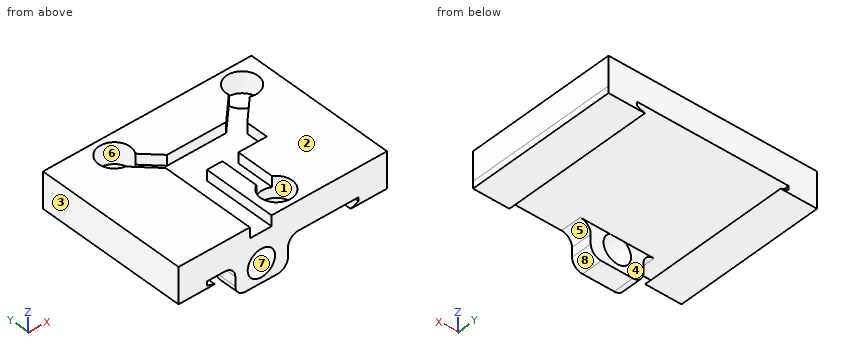
Autodesk Inventor part; units mm, degrees
ref_plane "YZ Plane" through (0, 0, 0) normal (1, 0, 0) x (0, 1, 0)
ref_plane "XZ Plane" through (0, 0, 0) normal (0, 1, 0) x (-1, 0, 0)
ref_plane "XY Plane" through (0, 0, 0) normal (0, 0, 1) x (1, 0, 0)
ref_plane "Work Plane1" through (52.5141, 202.7033, 6.4479) normal (0, 0, -1) x (0, 1, 0)
sketch "Sketch1" plane through (52.5141, 202.7033, 6.4479) normal (0, 0, -1) x (0, 1, 0)
  circle A0 centre (-59.8114, -30.5) radius 1.4 construction
  circle A1 centre (-38.8114, -18.3756) radius 1.4
  circle A2 centre (-38.8114, -42.6244) radius 1.4 construction
  circle A3 centre (41, 0) radius 1.65
  circle A4 centre (-9, 0) radius 1.65
  circle A5 centre (-9, 50) radius 1.65
  circle A6 centre (41, 50) radius 1.65
  circle A7 centre (16, 50) radius 1.65
  circle A8 centre (-9, 25) radius 1.65
  circle A9 centre (16, 0) radius 1.65
  circle A10 centre (41, 25) radius 1.65
  line L0 (80, 55) -> (-80, 55)
  line L1 (-80, 55) -> (-80, -55)
  line L2 (-80, -55) -> (80, -55)
  line L3 (80, -55) -> (80, 55)
  line L4 (-36.5, 0) -> (-36.5, -50)
  line L5 (-14, 0) -> (-36.5, 0)
  line L6 (-14, -5) -> (-14, 0)
  line L7 (72, -5) -> (-14, -5)
  line L8 (72, -50) -> (72, -5)
  line L9 (-36.5, -50) -> (72, -50)
  line L10 (-4, 45) -> (-4, 5)
  line L11 (36, 45) -> (-4, 45)
  line L12 (36, 5) -> (36, 45)
  line L13 (-4, 5) -> (36, 5)
  line L14 (-64.5989, -17.0433) -> (-64.5989, -57.0433) construction
  line L15 (-64.5989, -57.0433) -> (-34.5989, -57.0433) construction
  line L16 (-34.5989, -57.0433) -> (-34.5989, -17.0433) construction
  line L17 (-34.5989, -17.0433) -> (-64.5989, -17.0433) construction
  line L18 (-34.8114, -13.0433) -> (-63.8114, -13.0433)
  line L19 (-63.8114, -13.0433) -> (-63.8114, -52.6244)
  line L20 (-63.8114, -52.6244) -> (-34.8114, -52.6244)
  line L21 (-34.8114, -52.6244) -> (-34.8114, -13.0433)
  circle A11 centre (-59.8114, -30.5) radius 3
  circle A12 centre (-38.8114, -18.3756) radius 3
  circle A13 centre (-38.8114, -42.6244) radius 3 construction
  line L22 (-36.5, -35.1157) -> (-41.75, -35.1157) construction
  line L23 (-41.75, -35.1157) -> (-41.75, -38.5657) construction
  line L24 (-41.75, -38.5657) -> (-56.86, -38.5657) construction
  line L25 (-56.86, -38.5657) -> (-56.86, -35.1157) construction
  line L26 (-56.86, -35.1157) -> (-60.26, -35.1157) construction
  line L27 (-60.26, -35.1157) -> (-60.26, -52.0657) construction
  line L28 (-60.26, -52.0657) -> (-36.5, -52.0657) construction
  line L29 (-36.5, -52.0657) -> (-36.5, -35.1157) construction
  line L30 (-41.75, -28.3657) -> (-36.5, -28.3657) construction
  line L31 (-36.5, -28.3657) -> (-36.5, -25.0657) construction
  line L32 (-36.5, -25.0657) -> (-60.26, -25.0657) construction
  line L33 (-60.26, -25.0657) -> (-60.26, -28.3657) construction
  line L34 (-60.26, -28.3657) -> (-56.86, -28.3657) construction
  line L35 (-56.86, -28.3657) -> (-56.86, -27.0942) construction
  line L36 (-56.86, -27.0942) -> (-41.75, -27.0942) construction
  line L37 (-41.75, -27.0942) -> (-41.75, -28.3657) construction
  line L38 (-56.86, -35.1157) -> (-60.26, -35.1157) construction
  line L39 (-56.86, -38.5657) -> (-56.86, -35.1157) construction
  line L40 (-41.75, -38.5657) -> (-56.86, -38.5657) construction
  line L41 (-41.75, -35.1157) -> (-41.75, -38.5657) construction
  line L42 (-36.5, -35.1157) -> (-41.75, -35.1157) construction
  line L43 (-36.5, -35.05) -> (-36.5, -35.1157) construction
  line L44 (-36.5, -35.05) -> (-56.86, -35.05) construction
  line L45 (-36.5, -34.78) -> (-36.5, -35.05) construction
  line L46 (-36.5, -34.78) -> (-56.86, -34.78) construction
  line L47 (-36.5, -34.51) -> (-36.5, -34.78) construction
  line L48 (-36.5, -34.51) -> (-56.86, -34.51) construction
  line L49 (-36.5, -34.24) -> (-36.5, -34.51) construction
  line L50 (-36.5, -34.24) -> (-56.86, -34.24) construction
  line L51 (-36.5, -33.97) -> (-36.5, -34.24) construction
  line L52 (-36.5, -33.97) -> (-56.86, -33.97) construction
  line L53 (-36.5, -33.7) -> (-36.5, -33.97) construction
  line L54 (-36.5, -33.7) -> (-56.86, -33.7) construction
  line L55 (-36.5, -33.43) -> (-36.5, -33.7) construction
  line L56 (-36.5, -33.43) -> (-56.86, -33.43) construction
  line L57 (-36.5, -33.16) -> (-36.5, -33.43) construction
  line L58 (-36.5, -33.16) -> (-56.86, -33.16) construction
  line L59 (-36.5, -32.89) -> (-36.5, -33.16) construction
  line L60 (-36.5, -32.89) -> (-56.86, -32.89) construction
  line L61 (-36.5, -32.62) -> (-36.5, -32.89) construction
  line L62 (-36.5, -32.62) -> (-56.86, -32.62) construction
  line L63 (-36.5, -32.35) -> (-36.5, -32.62) construction
  line L64 (-36.5, -32.35) -> (-56.86, -32.35) construction
  line L65 (-36.5, -32.08) -> (-36.5, -32.35) construction
  line L66 (-36.5, -32.08) -> (-56.86, -32.08) construction
  line L67 (-36.5, -31.81) -> (-36.5, -32.08) construction
  line L68 (-36.5, -31.81) -> (-56.86, -31.81) construction
  line L69 (-36.5, -31.54) -> (-36.5, -31.81) construction
  line L70 (-36.5, -31.54) -> (-56.86, -31.54) construction
  line L71 (-36.5, -31.27) -> (-36.5, -31.54) construction
  line L72 (-36.5, -31.27) -> (-56.86, -31.27) construction
  line L73 (-36.5, -31) -> (-36.5, -31.27) construction
  line L74 (-36.5, -31) -> (-56.86, -31) construction
  line L75 (-36.5, -30.73) -> (-36.5, -31) construction
  line L76 (-36.5, -30.73) -> (-56.86, -30.73) construction
  line L77 (-36.5, -30.46) -> (-36.5, -30.73) construction
  line L78 (-36.5, -30.46) -> (-56.86, -30.46) construction
  line L79 (-36.5, -30.19) -> (-36.5, -30.46) construction
  line L80 (-36.5, -30.19) -> (-56.86, -30.19) construction
  line L81 (-36.5, -29.92) -> (-36.5, -30.19) construction
  line L82 (-36.5, -29.92) -> (-56.86, -29.92) construction
  line L83 (-36.5, -29.65) -> (-36.5, -29.92) construction
  line L84 (-36.5, -29.65) -> (-56.86, -29.65) construction
  line L85 (-36.5, -29.38) -> (-36.5, -29.65) construction
  line L86 (-36.5, -29.38) -> (-56.86, -29.38) construction
  line L87 (-36.5, -29.11) -> (-36.5, -29.38) construction
  line L88 (-36.5, -29.11) -> (-56.86, -29.11) construction
  line L89 (-36.5, -28.84) -> (-36.5, -29.11) construction
  line L90 (-36.5, -28.84) -> (-56.86, -28.84) construction
  line L91 (-36.5, -28.3657) -> (-36.5, -28.84) construction
  line L92 (-41.75, -28.3657) -> (-36.5, -28.3657) construction
  line L93 (-41.75, -27.0942) -> (-41.75, -28.3657) construction
  line L94 (-56.86, -27.0942) -> (-41.75, -27.0942) construction
  line L95 (-56.86, -28.3657) -> (-56.86, -27.0942) construction
  line L96 (-60.26, -28.3657) -> (-56.86, -28.3657) construction
  line L97 (-60.26, -35.1157) -> (-60.26, -28.3657) construction
  line L98 (-60.26, -25.0657) -> (-36.5, -25.0657) construction
  line L99 (-36.5, -25.0657) -> (-36.5, -52.0657) construction
  line L100 (-60.26, -52.0657) -> (-60.26, -25.0657) construction
  line L101 (-57.1632, -22.5233) -> (-33.4032, -22.5233) construction
  line L102 (-33.4032, -22.5233) -> (-33.4032, -49.5233) construction
  line L103 (-33.4032, -49.5233) -> (-57.1632, -49.5233) construction
  line L104 (-57.1632, -49.5233) -> (-57.1632, -22.5233) construction
  circle A14 centre (-38.8114, -42.6244) radius 3
  point P0 (-202.7033, -52.5141)
  point P1 (-56.7146, -27.9576)
  dimension "d0" = 4
  dimension "d2" = 4
  dimension "d3" = 4
  dimension "d4" = 6
  dimension "d5" = 6
  dimension "d6" = 6
  dimension "d10" = 10
extrude "Extrusion1" add sketch "Sketch1" along normal blind 4 contours L18 L21 L9 L4 A14 A12 | L4 A12 A14 L9 L21 L20 L19 L18
sketch "Sketch2" plane through (52.5141, 202.7033, 2.4479) normal (0, 0, -1) x (-1, 0, 0)
  circle A0 centre (42.6244, -38.8114) radius 3
  circle A1 centre (18.3756, -38.8114) radius 3
  circle A2 centre (30.5, -59.8114) radius 3
  line L0 (13.0433, -34.8114) -> (13.0433, -63.8114)
  line L1 (13.0433, -63.8114) -> (52.6244, -63.8114)
  line L2 (52.6244, -63.8114) -> (52.6244, -34.8114)
  line L3 (52.6244, -34.8114) -> (13.0433, -34.8114)
  point P0 (52.5141, -202.7033)
extrude "Extrusion2" add sketch "Sketch2" along normal blind 1.5 contours A0 | A1 | A2 | L3 L2 L1 L0
sketch "Sketch3" plane through (-0.1103, 138.8919, 6.4479) normal (0, -1, 0) x (1, 0, 0)
  line L0 (39.581, 0) -> (0, 0) construction
  line L1 (0, 0) -> (0, -5.5) construction
  line L2 (39.581, -5.5) -> (0, -5.5)
  line L3 (39.581, 0) -> (39.581, -5.5)
  line L4 (17.5087, -7.4479) -> (17.5087, -6.8479) construction
  line L5 (17.5087, -6.8479) -> (24.2587, -6.8479) construction
  line L6 (24.2587, -6.8479) -> (24.2587, -7.4479) construction
  line L7 (27.5587, -7.4479) -> (24.2587, -7.4479) construction
  line L8 (27.5587, -6.4479) -> (27.5587, -7.4479) construction
  line L9 (27.5587, -6.4479) -> (0.5587, -6.4479) construction
  line L10 (0.5587, -6.4479) -> (0.5587, -7.4479) construction
  line L11 (17.5087, -7.4479) -> (0.5587, -7.4479) construction
  line L12 (39.581, 0) -> (39.581, -5.5) construction
  line L13 (39.581, -5.5) -> (34.1825, -5.5)
  line L14 (34.1825, -5.5) -> (34.1825, -6.25)
  line L15 (34.8694, -6.8) -> (39.581, -6.8)
  line L16 (39.581, -6.8) -> (39.581, -5.5)
  line L17 (39.581, -6.8) -> (32.6714, -6.8)
  line L18 (32.6714, -6.8) -> (34.1825, -6.25)
  line L19 (12.6726, -5.5) -> (12.6726, -6.5)
  line L20 (0, 0) -> (0, -5.5) construction
  line L21 (0, -5.5) -> (5.3846, -5.5)
  line L22 (6.8957, -6.8) -> (0, -6.8)
  line L23 (0, -6.8) -> (0, -5.5)
  line L24 (6.8957, -6.8) -> (6.8957, -6.8)
  line L25 (0, -5.5) -> (39.581, -5.5)
  line L26 (6.8957, -6.8) -> (5.3846, -6.25)
  line L27 (5.3846, -6.25) -> (5.3846, -5.5)
  line L28 (5.9957, -5.5) -> (33.4957, -5.5) construction
  line L29 (33.4957, -5.5) -> (33.4957, -6.5) construction
  line L30 (33.4957, -6.5) -> (5.9957, -6.5) construction
  line L31 (5.9957, -6.5) -> (5.9957, -5.5) construction
  point P0 (8.981, -5.5)
  dimension "d42" = 1.3
  dimension "d43" = 110
  dimension "d45" = 0.75
  dimension "h1" = 0.75
  dimension "d47" = 110
  dimension "d48" = 27.5
  dimension "d49" = 1
  dimension "d50" = 0.9
  dimension "d51" = 0
extrude "Extrusion3" add sketch "Sketch3" against normal up to surface (29 mm away)
sketch "Sketch6" plane through (52.5141, 202.7033, 6.4479) normal (0, 0, 1) x (1, 0, 0)
  line L0 (-13.0433, -34.8114) -> (-13.0433, -63.8114)
  line L1 (-52.6244, -34.8114) -> (-13.0433, -34.8114)
  line L2 (-52.6244, -63.8114) -> (-52.6244, -34.8114)
  line L3 (-13.0433, -63.8114) -> (-52.6244, -63.8114)
  line L4 (-23.5962, -45.8071) -> (-17.5454, -39.7563)
  line L5 (-17.5454, -39.7563) -> (-19.6668, -37.635)
  line L6 (-19.6668, -37.635) -> (-25.7175, -43.6858)
  line L7 (-25.7175, -43.6858) -> (-23.5962, -45.8071)
  line L8 (-23.5962, -45.8071) -> (-19.6668, -37.635) construction
  line L9 (-17.5454, -39.7563) -> (-25.7175, -43.6858) construction
  line L10 (-39.0797, -45.8071) -> (-43.9064, -40.9803)
  line L11 (-43.9064, -40.9803) -> (-41.7851, -38.859)
  line L12 (-41.7851, -38.859) -> (-36.9583, -43.6858)
  line L13 (-36.9583, -43.6858) -> (-39.0797, -45.8071)
  line L14 (-39.0797, -45.8071) -> (-41.7851, -38.859) construction
  line L15 (-43.9064, -40.9803) -> (-36.9583, -43.6858) construction
  line L16 (-25.7175, -43.6858) -> (-36.9583, -43.6858)
  line L17 (-23.5962, -45.8071) -> (-23.5962, -49.9899)
  line L18 (-23.5962, -49.9899) -> (-39.0797, -49.9899)
  line L19 (-39.0797, -49.9899) -> (-39.0797, -45.8071)
  line L20 (-32.0216, -49.9899) -> (-28.9927, -49.9899)
  line L21 (-28.9927, -49.9899) -> (-28.9927, -57.6065)
  line L22 (-28.9927, -57.6065) -> (-32.0216, -57.6065)
  line L23 (-32.0216, -57.6065) -> (-32.0216, -49.9899)
  line L24 (-39.0797, -45.8071) -> (-39.0797, -49.9899)
  line L25 (-45.7287, -63.8114) -> (-45.7287, -34.8114) construction
  line L26 (-39.0797, -49.9899) -> (-34.9564, -49.9899)
  line L27 (-34.9564, -49.9899) -> (-34.9564, -63.8114)
  line L28 (-34.9564, -63.8114) -> (-39.0797, -63.8114)
  line L29 (-39.0797, -63.8114) -> (-39.0797, -49.9899)
  point P0 (-52.5141, -202.7033)
  point P1 (-21.6315, -41.7211)
  point P2 (-40.4324, -42.333)
  dimension "d35" = 3
  dimension "d36" = 3
  dimension "d37" = 45
  dimension "d38" = 0
extrude "Extrusion6" cut sketch "Sketch6" against normal blind 2 contours L3 L29 L18 L27 | L18 L19 L13 L16 L7 L17 | L18 L21 L22 L23 | L10 L11 L12 L13 | L6 L5 L4 L7
sketch "Sketch7" plane through (-0.1103, 138.8919, 6.4479) normal (0, -1, 0) x (0, 0, 1)
  line L0 (-11.273, -20.7778) -> (-5.5, -20.7778)
  line L1 (-5.5, -20.7778) -> (-5.5, -10.7778)
  line L2 (-5.5, -10.7778) -> (-11.273, -10.7778)
  line L3 (-11.273, -10.7778) -> (-11.273, -20.7778)
  line L4 (-5.5, -34.1825) -> (-5.5, -5.3846)
  point P0 (-6.8, -32.6714)
  dimension "d53" = 10
extrude "Extrusion7" add sketch "Sketch7" against normal blind 4
fillet "Fillet1" radius 2 4 edges at (10.6675, 140.8919, -4.8251) (20.6675, 140.8919, -4.8251) (10.6675, 140.8919, 0.9479) (20.6675, 140.8919, 0.9479)
sketch "Sketch8" plane through (-0.1103, 138.8919, 6.4479) normal (0, -1, 0) x (0, 0, 1)
  line L0 (0, 0) -> (-6.8, 0)
  line L1 (0, 0) -> (-6.8, 0)
  circle A0 centre (-7.6471, -15.7336) radius 2.6
  line L2 (-6.8, 0) -> (-6.8, 0)
  point P0 (-6.4479, -0.1103)
  dimension "d58" = 5.2
extrude "Extrusion8" cut sketch "Sketch8" against normal up to surface (4 mm away)
equation "\"d45\" = h1"
properties part number "cellSTORM_v5_chiptray_old_0"
Build history of the part. All positions in model axes, mm. Face numbers are marked on the shaded views. A direction names the side the tool comes from. Round coordinates to 2 decimals unless told otherwise and drop trailing zeros. Write each loop counter-clockwise with the first axis right and the second up, starting at its lowest first coordinate (ties: lowest second). Pieces come first, ordered by that corner, then holes. Notation, with made-up numbers: (15.5, 74) -> (69.5, 74) arc R28 cw to (69.5, 96) -> close; hole circle Ø9 at (71.5, 44). An arc over 180 degrees is marked (long way). Use one line per item in the form item = value.
Q1. Band-saw the part on C-C, the plane x = 20. Write the cut outline in (y, z), then the cut area to 3 significant figures.
Conclusion:
outline = (138.89, -4.32) -> (142.89, -4.32) -> (142.89, 0.95) -> (167.89, 0.95) -> (167.89, 6.45) -> (159.02, 6.45) -> (159.02, 4.45) -> (152.71, 4.45) -> (152.71, 6.45) -> (145.12, 6.45) -> (145.12, 2.45) -> (140.67, 2.45) -> (140.67, 6.45) -> (138.89, 6.45) -> close
area = 150 mm²
Q2. Drop flat-ended pins along their axis: P1, Ø8, axis at x = 14, y = 145, coming from the -Z side; P2, Ø14.5, axis at x = 20.5, y = 160, coming from the -Z side; P3, Ø4, axis at x = 15.62, z = -1.2, coming from the +Y side; P4, Ø1.8, axis at x = 20.5, y = 143, coming from the +Z side. Give the stop position or say it passes through.
Conclusion:
P1 = -4.83
P2 = 0.95
P3 = through
P4 = 2.45
Q3. Two-plate mould, pull along X, no slides. Class the marked faces 1, 2 and 3: released by +X, released by -X, zero draft, split by the parting line, or undercut.
Conclusion:
face_1 = undercut
face_2 = zero draft
face_3 = released by -X
Q4. Drill centre lines: L1, parallel to X at y = 146.75, z = 6; L2, parallel to Y at x = 12.5, z = 6.25; L3, parallel to X at y = 159.25, z = 5. Where is each one in solid material? Low to high.
Conclusion:
L1 = -0.11 to 13.43, 17.56 to 20.49, 23.52 to 39.47
L2 = 138.89 to 157.83, 162.07 to 162.41, 165.37 to 167.89
L3 = -0.11 to 11.08, 15.32 to 27.03, 31.27 to 39.47
Q5. Band-saw the part on B-B, the plane y = 151.5. Write the cut outline in (x, z).
Conclusion:
outline = (-0.11, -0.35) -> (6.79, -0.35) -> (5.27, 0.2) -> (5.27, 0.95) -> (34.07, 0.95) -> (34.07, 0.2) -> (32.56, -0.35) -> (39.47, -0.35) -> (39.47, 6.45) -> (23.52, 6.45) -> (23.52, 4.45) -> (20.49, 4.45) -> (20.49, 6.45) -> (17.56, 6.45) -> (17.56, 4.45) -> (13.43, 4.45) -> (13.43, 6.45) -> (-0.11, 6.45) -> close
Q6. Band-saw the part on A-A, the plane z = 5.25. Write the cut outline in (x, y).
Conclusion:
outline = (-0.11, 138.89) -> (13.43, 138.89) -> (13.43, 156.9) -> (9.4, 160.93) arc R3 cw (long way) to (12.37, 162.2) -> (15.56, 159.02) -> (26.8, 159.02) -> (31.18, 163.4) arc R3 cw (long way) to (33.1, 161.08) -> (28.92, 156.9) -> (28.92, 152.71) -> (23.52, 152.71) -> (23.52, 145.49) arc R3 cw (long way) to (20.49, 145.48) -> (20.49, 152.71) -> (17.56, 152.71) -> (17.56, 138.89) -> (39.47, 138.89) -> (39.47, 167.89) -> (-0.11, 167.89) -> close
Q7. Tool access for the marked faces 4, 5, 6, 7 and 8: list every direction of +Z, -Z, +X, -X, +Y, -Y with a clear straight run to the whole face (end or side of a thin tool).
Conclusion:
face_4 = -Z, +Y
face_5 = -Z, +Y, -Y
face_6 = +Z
face_7 = -Y
face_8 = -Z, +X, +Y, -Y
Q8. Band-saw the part on D-D, the plane y = 144.25. Write the cut outline in (x, z).
Conclusion:
outline = (-0.11, -0.35) -> (6.79, -0.35) -> (5.27, 0.2) -> (5.27, 0.95) -> (34.07, 0.95) -> (34.07, 0.2) -> (32.56, -0.35) -> (39.47, -0.35) -> (39.47, 6.45) -> (24.69, 6.45) -> (24.69, 2.45) -> (19.34, 2.45) -> (19.34, 6.45) -> (17.56, 6.45) -> (17.56, 4.45) -> (13.43, 4.45) -> (13.43, 6.45) -> (-0.11, 6.45) -> close
